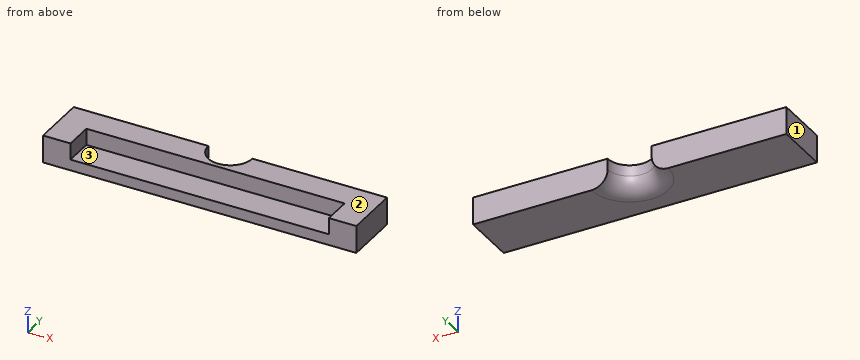
from build123d import *

# Parameters (mm, degrees)
SKETCH1_W           = 57
SKETCH1_H           = 10
BOSS_EXTRUDE1_DEPTH = 5
SKETCH2_W           = 47
SKETCH2_H           = 5.162319645
CUT_EXTRUDE1_DEPTH  = 3
CUT_EXTRUDE2_DEPTH  = 6
FILLET1_R           = 3


with BuildPart() as part:
    # Sketch1 → Boss-Extrude1 (new body)
    with BuildSketch(Plane.XY):
        with Locations((28.5, -5)):
            Rectangle(SKETCH1_W, SKETCH1_H)
    extrude(amount=BOSS_EXTRUDE1_DEPTH)

    # Sketch2 → Cut-Extrude1 (cut)
    with BuildSketch(Plane.XY.offset(5)):
        with Locations((28.5, -7.418840177)):
            Rectangle(SKETCH2_W, SKETCH2_H)
    extrude(amount=-CUT_EXTRUDE1_DEPTH, mode=Mode.SUBTRACT)

    # Sketch3 → Cut-Extrude2 (cut, through all)
    with BuildSketch(Plane(origin=(0, 0, 0), x_dir=(-1, 0, 0), z_dir=(0, 0, -1))):
        with BuildLine():
            Line((-32.5, 0), (-24.5, 0))
            ThreePointArc((-24.5, 0), (-28.5, -4), (-32.5, 0))
        make_face()
    extrude(amount=-CUT_EXTRUDE2_DEPTH, mode=Mode.SUBTRACT)

    # Fillet1
    fillet1_edges = [part.edges().sort_by_distance(p)[0] for p in [
        (28.5, -4, 0),
    ]]
    fillet(fillet1_edges, radius=FILLET1_R)


solid = part.part
The listing builds one solid part. Answer for the finished solid, in the listing's coordinates (mm). Face numbers are marked on the shaded views. Round coordinates to 2 decimals unless told otherwise and drop trailing zeros. Loops run counter-clockwise (first coordinate to the right, second up) from the corner with the lowest first, then second, coordinate; pieces in that order, holes last. Notation, with made-up numbers: M 84,2 L 95,2 A32 cw 95,40 Z; hole C 23,13.5 d7. An arc over 180 degrees is marked long. Return JSON: item names as keys, results as strings.
Q1. Find the intervals of material crossed by line 1 along X through (y, z) = (-8.5, 4.35); line 2 along Y through (x, z) = (48, 3.8); line 3 along Z through (x, y) = (24.5, -5.75), in increasing order. Write a range as from..to.
Results list:
{"line 1": "x = 0..5, 52..57", "line 2": "y = -4.84..0", "line 3": "z = 0..2"}
Q2. Each of these flat-tipped pins is pushed along its axis until it touches: pin 1 Ø2.5 at (x, z) = (26, 4) entering from -Y; pin 2 Ø1.5 at (x, y) = (29.5, -6.5) entering from +Z. Where does it stop, or does it pass through?
Results list:
{"pin 1": "stops at y = -4.84", "pin 2": "stops at z = 2"}
Q3. Find section C-C, the plane z = 4.35. Determine the outline of the cut face in (x, y), plus the area to 3 significant figures.
Results list:
{"outline": "M 0,-10 L 5,-10 L 5,-4.84 L 52,-4.84 L 52,-10 L 57,-10 L 57,0 L 32.5,0 A4 cw 24.5,0 L 0,0 Z", "area": "302 mm2"}
Q4. Find section A-A, the plane y = -8.5. Determine the outline of the cut face in (x, z).
Results list:
{"outline": "M 0,0 L 57,0 L 57,5 L 52,5 L 52,2 L 5,2 L 5,5 L 0,5 Z"}
Q5. Find section B-B, the plane x = 20.5. Determine the outline of the cut face in (y, z), plus the area to 3 significant figures.
Results list:
{"outline": "M -10,0 L 0,0 L 0,5 L -4.84,5 L -4.84,2 L -10,2 Z", "area": "34.5 mm2"}
Q6. Find section D-D, the plane x = 28.5. Determine the outline of the cut face in (y, z).
Results list:
{"outline": "M -10,0 L -7,0 A3 ccw -4,3 L -4,5 L -4.84,5 L -4.84,2 L -10,2 Z"}
Q7. The mould has two halves that part along X. Classify the marked faces 1, 2 and 3: released by +X, released by -X, zero draft, split by the parting line, or undercut.
Results list:
{"face 1": "released by -X", "face 2": "zero draft", "face 3": "undercut"}
